CAD build for the part. Positions are in the model's coordinates, mm. A direction names the side the tool comes from. Give positions to 0.01 mm unless a question says otherwise; leave off trailing zeros. Loops run counter-clockwise (first coordinate to the right, second up) from the corner with the lowest first, then second, coordinate; pieces in that order, holes last.
Item 1: Saw through at D-D on y = -3. Give the number of separate pieces and of enclosed holes in the cut face, plus the area to 3 significant figures.
Item 2: Mould opens along Z. For faces 1 (the cylindrical face through (-17.89, -2.44, -12.04)), 2 (the flat face through (15, -5, -3)), 3 (the flat face through (-14, -3, 9)), 4 (the flat face through (0, -3, 15)) say: released by +Z, released by -Z, zero draft, split by the parting line, or undercut.
Item 3: Drop flat-ended pins along their axis: P1, Ø3.5, axis at x = 17.5, y = -2.5, coming from the +Z side; P2, Ø1.8, axis at y = -2.5, z = 7.5, coming from the +X side; P3, Ø1.5, axis at y = -2, z = 10.5, coming from the -X side. Give the stop position or say it passes through.
Item 4: Saw through at B-B on z = -7. Give the cut face in (x, y), plus the area to 3 significant figures.
Item 5: Which spindle directions (+Z, -Z, +X, -X, +Y, -Y) get a long thin tool onto all of the face, cutting with end or side? Do faces 5 (the flat face through (0, -3, -15)), 6 (the flat face through (15, -5, 3)), 7 (the flat face through (-14, -3, -9)). Say none if no direction does.
Item 6: Saw through at C-C on y = -6. Give the cut face in (x, z), plus the area to 3 significant figures.
Item 7: Probe probe 1 along Z at (x, y) = (17, -0.5); probe 2 along X at (y, z) = (-3.5, 0.5); probe 3 along Y at (x, z) = (16.5, -11.35). List the from-to ranges inside material, lowest first.
Item 8: Saw through at A-A on z = -0.75. Give the cut face in (x, y), plus the area to 3 significant figures.
from build123d import *

# Parameters (mm, degrees)
F0_W     = 7
F0_H     = 6
F1_DEPTH = 7
F2_R     = 1.75
F3_DEPTH = 30.001


# Not quite as in the source:
# - a feature names something its author has since deleted; it is built from what else it names


with BuildPart() as f1:
    # F0 (on Front) → F1 (new body)
    with BuildSketch(Plane.XZ):
        with Locations((16.5, 12)):
            Rectangle(F0_W, F0_H)
        with Locations((16.5, -12)):
            Rectangle(F0_W, F0_H)
        with Locations((16.5, 0)):
            Rectangle(F0_W, F0_H)
        with Locations((-16.5, 12)):
            Rectangle(F0_W, F0_H)
        with Locations((-16.5, 0)):
            Rectangle(F0_W, F0_H)
        with Locations((-16.5, -12)):
            Rectangle(F0_W, F0_H)
        Polygon((13, 9), (13, 15), (-13, 15), (-13, 9), (-13, 3), (-13, -3), (-13, -9), (-13, -15), (13, -15), (13, -9), (13, -3), (13, 3), align=None)
    extrude(amount=F1_DEPTH)

    # F2 (on face) → F3 (cut, through all)
    with BuildSketch(Plane(origin=(0, 0, -15), x_dir=(1, 0, 0), z_dir=(0, 0, -1))):
        with Locations((-16.5, 3.5)):
            Circle(F2_R)
        with BuildLine():
            Line((-20, 0), (-16.5, 0))
            ThreePointArc((-16.5, 0), (-18.9748737342, 1.0251262658), (-20, 3.5))
            Line((-20, 3.5), (-20, 0))
        make_face()
        with BuildLine():
            ThreePointArc((-20, 3.5), (-18.9748737342, 5.9748737342), (-16.5, 7))
            Line((-16.5, 7), (-20, 7))
            Line((-20, 7), (-20, 3.5))
        make_face()
        with BuildLine():
            Line((20, 7), (16.5, 7))
            ThreePointArc((16.5, 7), (18.9748737342, 5.9748737342), (20, 3.5))
            Line((20, 3.5), (20, 7))
        make_face()
        with BuildLine():
            ThreePointArc((20, 3.5), (18.9748737342, 1.0251262658), (16.5, 0))
            Line((16.5, 0), (20, 0))
            Line((20, 0), (20, 3.5))
        make_face()
        with Locations((16.5, 3.5)):
            Circle(F2_R)
    extrude(amount=-F3_DEPTH, mode=Mode.SUBTRACT)


solid = f1.part
Results below:
1. separate pieces: 7
1. enclosed holes: 0
1. area: 910 mm2
2. face 1: zero draft
2. face 2: undercut
2. face 3: undercut
2. face 4: released by +Z
3. P1: stops at z = 15
3. P2: stops at x = 13
3. P3: stops at x = -19.92
4. outline: (-13, -7) - (13, -7) - (13, 0) - (-13, 0) - close
4. area: 182 mm2
5. face 5: -Z, +X, -X, +Y, -Y
5. face 6: +X, +Y, -Y
5. face 7: -X, +Y, -Y
6. outline: (-18.95, -15) - (18.95, -15) - (18.95, -9) - (13, -9) - (13, -3) - (18.95, -3) - (18.95, 3) - (13, 3) - (13, 9) - (18.95, 9) - (18.95, 15) - (-18.95, 15) - (-18.95, 9) - (-13, 9) - (-13, 3) - (-18.95, 3) - (-18.95, -3) - (-13, -3) - (-13, -9) - (-18.95, -9) - close
6. area: 994 mm2
7. probe 1: z = -15 to -9, -3 to 3, 9 to 15
7. probe 2: x = -20 to -18.25, -14.75 to 14.75, 18.25 to 20
7. probe 3: y = -7 to -5.25, -1.75 to 0
8. outline: (-16.5, -7) - (16.5, -7) arc R3.5 ccw to (16.5, 0) - (-16.5, 0) arc R3.5 ccw to start; hole circle Ø3.5 at (-16.5, -3.5); hole circle Ø3.5 at (16.5, -3.5)
8. area: 250 mm2
